The model under review builds one solid part; all positions refer to its coordinate system, in mm. A direction names the side the tool comes from. Coordinates: 2 decimals unless noted, no trailing zeros. Write each loop counter-clockwise with the first axis right and the second up, starting at its lowest first coordinate (ties: lowest second). Pieces come first, ordered by that corner, then holes. Notation, with made-up numbers: (78.5, -21.75) - (126.5, -21.75) arc R35 ccw to (126.5, 14.25) - close; hole circle Ø10 at (46.5, 64.5). An arc over 180 degrees is marked (long way). Return JSON: item names as keys, results as strings. Group by question number.
(1) For pin 1 Ø8 at (x, y) = (-22, -16) entering from -Z; pin 2 Ø8 at (x, z) = (-18, 43) entering from -Y; pin 3 Ø12 at (x, y) = (14, 8) entering from +Z, all flat-tipped, find the tip position at first contact; note any pin that passes through.
(2) To check wall thickness, follow L1, parallel to Z at x = -27.5, y = 13.5; L2, parallel to Z at x = -4, y = -0.5; L3, parallel to Y at x = 22, z = 59.5. State the ranges of each line that lie inside material, in increasing order. Write a range as from..to.
(3) We need section C-C on z = 27.5. State the section outline as (x, y) points.
(4) Tool access review of faces 1 (the face through (1, 11, 1.588)), 2 (the face through (1, 10, 0)): name each direction out of +Z, -Z, +X, -X, +Y, -Y from which nothing blocks a thin tool from reaching the whole face with its end or side.
(5) We need section B-B on y = 10. State the section outline as (x, z) points, then the cut area to 3 significant figures.
```python
from build123d import *

# Parameters (mm, degrees)
F1_DEPTH = 57.94375


with BuildPart() as f1:
    # F0 (on Right) → F1 (new body, symmetric)
    with BuildSketch(Plane.YZ):
        with BuildLine():
            Line((3.503151, 0), (15.875, 0))
            Line((15.875, 0), (15.875, 1.5875))
            Line((15.875, 1.5875), (5.163465, 1.5875))
            ThreePointArc((5.163465, 1.5875), (2.131531, 2.358085), (-0.164541, 4.482815))
            Line((-0.164541, 4.482815), (-39.0525, 64.457974))
            Line((-39.0525, 64.457974), (-40.64, 64.457974))
            Line((-40.64, 64.457974), (-1.868347, 2.963333))
            ThreePointArc((-1.868347, 2.963333), (0.435809, 0.789972), (3.503151, 0))
        make_face()
    extrude(amount=F1_DEPTH, both=True)


solid = f1.part
```
Ans:
{
 "1": {"pin 1": "z = 19.03", "pin 2": "y = -29.63", "pin 3": "z = 2.43"},
 "2": {"L1": "0..1.59", "L2": "1.42..5", "L3": "-37.51..-35.84"},
 "3": {"outline": "(-57.94, -17.34) - (57.94, -17.34) - (57.94, -15.09) - (-57.94, -15.09) - close"},
 "4": {"face 1": "+Z, +X, -X, +Y", "face 2": "-Z, +X, -X, +Y, -Y"},
 "5": {"outline": "(-57.94, 0) - (57.94, 0) - (57.94, 1.59) - (-57.94, 1.59) - close", "area": "184 mm²"}
}
